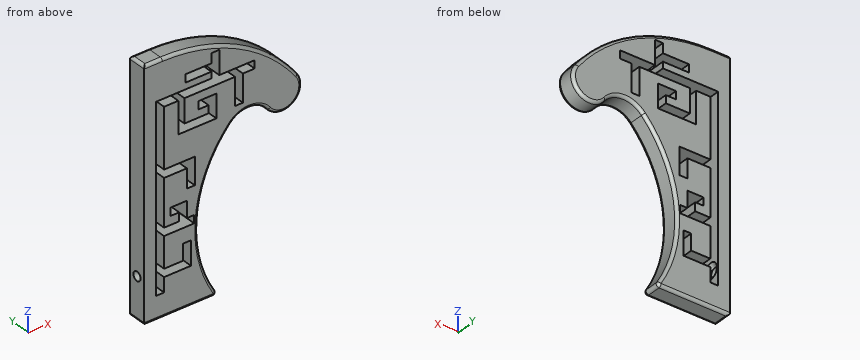
from build123d import *

# Parameters (mm, degrees)
BOSS_EXTRUDE1_DEPTH = 10
FILLET1_R           = 1.5


with BuildPart() as part:
    # Sketch1 → Boss-Extrude1 (new body)
    with BuildSketch(Plane(origin=(0, 0, 0), x_dir=(1, 0, 0), z_dir=(0, 1, 0))):
        with BuildLine():
            Line((0, 132), (0, 0))
            Line((0, 0), (9.806899205, 0))
            ThreePointArc((9.806899205, 0), (50.833969992, 9.773283566), (83.048530962, 36.993857965))
            ThreePointArc((83.048530962, 36.993857965), (81.000199646, 50.92844911), (67.049362803, 48.993857965))
            ThreePointArc((67.049362803, 48.993857965), (57.146860922, 43.813297067), (46.819761712, 48.085155754))
            ThreePointArc((46.819761712, 48.085155754), (29.029737588, 88.873903236), (40, 132))
            Line((40, 132), (0, 132))
        make_face()
        Polygon((6.5, 20.67103065), (6.5, 119.400046722), (10.75, 119.400046722), (10.75, 111.574341839), (25.276432371, 111.574341839), (25.276432371, 107.324341839), (25.276432371, 98.607245151), (21.026432371, 98.607245151), (21.026432371, 107.324341839), (10.75, 107.324341839), (10.75, 90.692748994), (26.995661983, 90.692748994), (26.995661983, 86.442748994), (23.122830992, 86.442748994), (23.122830992, 77.602272136), (18.872830992, 77.602272136), (14.275783025, 77.602272136), (14.275783025, 81.852272136), (18.872830992, 81.852272136), (18.872830992, 86.442748994), (10.75, 86.442748994), (10.75, 61.130194379), (23.055943787, 61.130194379), (23.055943787, 71.449300242), (27.305943787, 71.449300242), (27.305943787, 61.130194379), (27.305943787, 56.880194379), (10.75, 56.880194379), (10.75, 24.92103065), (18.412851079, 24.92103065), (18.412851079, 42.066790132), (21.749945206, 42.066790132), (39.003105081, 42.066790132), (39.003105081, 37.816790132), (39.003105081, 29.408846891), (34.753105081, 29.408846891), (29.22963894, 29.408846891), (29.22963894, 33.658846891), (34.753105081, 33.658846891), (34.753105081, 37.816790132), (21.749945206, 37.816790132), (21.749945206, 24.92103065), (49.043283634, 24.92103065), (49.043283634, 39.766503131), (53.293283634, 39.766503131), (53.293283634, 24.92103065), (59.608702719, 24.92103065), (59.608702719, 20.67103065), (40.548717705, 20.67103065), (40.548717705, 7.79221883), (36.298717705, 7.79221883), (36.298717705, 12.986428014), (22.249875285, 12.986428014), (22.249875285, 17.236428014), (36.298717705, 17.236428014), (36.298717705, 20.67103065), (10.75, 20.67103065), align=None, mode=Mode.SUBTRACT)
    extrude(amount=BOSS_EXTRUDE1_DEPTH)

    # Fillet1
    fillet1_edges = [part.edges().sort_by_distance(p)[0] for p in [
        (0, 5, 0),
        (0, 5, -132),
        (40, 5, -132),
        (4.903449602, 10, 0),
        (50.833969992, 10, -9.773283566),
        (81.000199646, 10, -50.92844911),
        (57.146860922, 10, -43.813297067),
        (29.029737588, 10, -88.873903236),
        (20, 10, -132),
        (20, 0, -132),
        (29.029737588, 0, -88.873903236),
        (57.146860922, 0, -43.813297067),
        (81.000199646, 0, -50.92844911),
        (50.833969992, 0, -9.773283566),
        (4.903449602, 0, 0),
    ]]
    fillet(fillet1_edges, radius=FILLET1_R)

    # Sketch5 → CSK for #8 Flat Head Machine Screw2 (revolve, cut)
    with BuildSketch(Plane(origin=(6.5, 5, -109.449341839), x_dir=(0, 0, -1), z_dir=(0, 1, 0))):
        Polygon((0, 0), (0, 11.476584928), (2.45745, 10), (2.45745, 2.02344051), (4.2164, 0), align=None)
    revolve(axis=Axis((12.85, 5, -109.449341839), (-1, 0, 0)), mode=Mode.SUBTRACT)


solid = part.part
The model under review builds one solid part; all positions refer to its coordinate system, in mm. Coordinates: 2 decimals unless noted, no trailing zeros. Put each result on its own line as item: value.
1) Wall thickness on probe 1 along X at (y, z) = (2.75, -102); probe 2 along Z at (x, y) = (11, 5.75); probe 3 along X at (y, z) = (2, -80.5): over which ranges is each line inside the solid? List them lowest first. Write a range as [from, to].
Computed:
probe 1: x = [0, 6.5], [10.75, 21.03], [25.28, 29.22]
probe 2: z = [-132, -111.57], [-107.32, -90.69], [-86.44, -61.13], [-56.88, -24.92], [-20.67, -0.01]
probe 3: x = [0, 6.5], [10.75, 14.28], [23.12, 30.23]
2) Clearance check with flat-ended pins moving along their axes: pin 1 Ø5 at (y, z) = (3.5, -56.5) entering from +X; pin 2 Ø5 at (y, z) = (7, -35.5) entering from +X; pin 3 Ø3 at (y, z) = (7, -89) entering from +X. State where each tip first meets the part, or that it passes through.
Computed:
pin 1: stops at x = 41.98
pin 2: stops at x = 83.7
pin 3: stops at x = 29.16
3) Add section A-A on x = 30.5. State how many separate pieces and enclosed holes the cut face has, then the cut area to 3 significant figures.
Computed:
separate pieces: 6
enclosed holes: 0
area: 813 mm2
